```python
from build123d import *

# Parameters (mm, degrees)
SKETCH5_R               = 12.7
SKETCH6_R               = 12.7
BOSS_EXTRUDE3_DEPTH     = 406.4
SKETCH7_R               = 12.7
BOSS_EXTRUDE4_DEPTH     = 203.2
SKETCH9_R               = 12.065
CUT_EXTRUDE2_DEPTH      = 6.35
SKETCH10_R              = 12.7
CUT_EXTRUDE3_DEPTH      = 462.222817168
CUT_EXTRUDE3_DEPTH_BACK = 462.222817168


with BuildPart() as part:
    # Sweep1: sweep along a path in Sketch4
    with BuildLine(Plane.XY) as sweep1_path:
        ThreePointArc((-38.874671546, 79.949796199), (-75.907697444, 46.273442371), (-88.87582946, -2.072905643))
    # Sketch5 → Sweep1 (sweep)
    with BuildSketch(Plane(origin=(0, 0, 0), x_dir=(1, 0, 0), z_dir=(0, 1, 0))):
        with Locations((-88.87582946, 0)):
            Circle(SKETCH5_R)
    sweep(path=sweep1_path.line)

    # Sketch6 → Boss-Extrude3 (add)
    with BuildSketch(Plane(origin=(0, 0, 0), x_dir=(0, 0, -1), z_dir=(0.8993227918843839, 0.43728539421901275, 0))):
        with Locations(Location((0, 88.87582946, 0), (0, 0, 180))):
            Circle(SKETCH6_R)
    extrude(amount=BOSS_EXTRUDE3_DEPTH)

    # Sketch7 → Boss-Extrude4 (add)
    with BuildSketch(Plane(origin=(0, 0, 0), x_dir=(-0.9997281154099812, -0.023317273828803834, 0), z_dir=(0.023317273828803834, -0.9997281154099812, 0))):
        with Locations((88.87582946, 0)):
            Circle(SKETCH7_R)
    extrude(amount=BOSS_EXTRUDE4_DEPTH)

    # Sketch9 → Cut-Extrude2 (cut)
    with BuildSketch(Plane(origin=(0, 0, -12.7), x_dir=(-1, 0, 0), z_dir=(0, 0, -1))):
        with Locations((76.269889492, 46.494235168)):
            Circle(SKETCH9_R)
    extrude(amount=-CUT_EXTRUDE2_DEPTH, mode=Mode.SUBTRACT)

    # Sweep2: sweep along a path in Sketch11
    with BuildLine(Plane.XY) as sweep2_path:
        Line((-84.113595449, -205.217095104), (-28.578350384, -319.431089673))
    # Sketch10 → Sweep2 (sweep)
    with BuildSketch(Plane(origin=(4.738070042, -203.144753051, 0), x_dir=(-0.9997281154099812, -0.023317273828803834, 0), z_dir=(0.023317273828803834, -0.9997281154099812, 0))):
        with Locations((88.87582946, 0)):
            Circle(SKETCH10_R)
    sweep(path=sweep2_path.line)

    # Sketch12 → Cut-Extrude3 (cut, two sides: drawn at the far end of the back side and taken through both)
    with BuildSketch(Plane.XY.offset(-CUT_EXTRUDE3_DEPTH_BACK)):
        Polygon((-41.274897449, -319.727219051), (-20.504520989, -309.627861689), (-15.881803318, -319.134960295), align=None)
    extrude(amount=CUT_EXTRUDE3_DEPTH + CUT_EXTRUDE3_DEPTH_BACK, mode=Mode.SUBTRACT)


solid = part.part
```
Design review of the part built by this model. Coordinates are the model's own, in mm. A direction names the side the tool comes from. Coordinates: 2 decimals unless noted, no trailing zeros.
Q1. The part is to be moulded in two halves that separate along X. For faces 4 (the face through (142.988, 164.11, 12.114)), 5 (the face through (-31.033, -314.747, -0.176)), 6 (the face through (-76, 47, -6.35)), 7 (the face through (-68.961, 56.093, -8.864)), say which applies: +X half, -X half, draft (parallel to the pull), parting line (faces both ways), or undercut.
Reported:
face 4: parting line
face 5: +X half
face 6: undercut
face 7: undercut
Q2. Tool access review of faces 1 (the face through (-98.626, -102.505, -3.815)), 2 (the face through (-81.1, 35.44, -8.86)), 3 (the face through (326.7, 257.48, -0.18)): name each direction out of +Z, -Z, +X, -X, +Y, -Y from which nothing blocks a thin tool from reaching the whole face with its end or side.
Reported:
face 1: none
face 2: -Z
face 3: +Z, -Z, +X, +Y
Q3. For pin 1 (12 mm diameter, centred on y = 90, z = -2, fed in from +X); pin 2 (12 mm diameter, centred on x = 149.5, z = 6, fed in from -Y); pin 3 (2 mm diameter, centred on y = -222.5, z = -6.5, fed in from +X), all flat-tipped, find the tip position at first contact; note any pin that passes through.
Reported:
pin 1: stops at x = 23
pin 2: stops at y = 155.27
pin 3: stops at x = -63.94
Q4. To check wall thickness, follow line 1 (Y direction, x = -24.5, z = -1); line 2 (Y direction, x = 78, z = 6); line 3 (Y direction, x = 306.5, z = -6.5). State the ranges of each line that lie inside material, in increasing order.
Reported:
line 1: y = -311.57 to -301.49, 72.83 to 100.99
line 2: y = 124.31 to 149.2
line 3: y = 235.73 to 259.99
